The model under review builds one solid part; all positions refer to its coordinate system, in mm. A direction names the side the tool comes from. Coordinates: 2 decimals unless noted, no trailing zeros. Write each loop counter-clockwise with the first axis right and the second up, starting at its lowest first coordinate (ties: lowest second). Pieces come first, ordered by that corner, then holes.
1) For P1, Ø3.5, axis at x = 171.5, z = 59.5, coming from the +Y side; P2, Ø4, axis at x = 127.5, y = 41, coming from the -Z side; P3, Ø2.5, axis at x = 55, y = 4.5, coming from the -Z side, all flat-tipped, find the tip position at first contact; note any pin that passes through.
2) For line 1 (Z direction, x = 172, y = 4.55); line 2 (X direction, y = 112, z = 12.5); line 3 (Z direction, x = 150, y = 63.5), list the stretches that pass through material, from the lowest coordinate up.
3) Add section C-C, the plane z = 107. State the section outline as (x, y) points.
4) Add section B-B, the plane y = 11. State the section outline as (x, z) points.
5) Machinability: for faces 4 (the flat face through (165, 5.5, 60)), 5 (the flat face through (110, 2.5, 60)), 6 (the flat face through (111, 2, 0)), 7 (the flat face through (224, 58, 61)), 8 (the flat face through (110.47, 137.92, 18.76)), which of the approach directions +Z, -Z, +X, -X, +Y, -Y give a long, thin tool a straight path to every point of the face, cutting with its end or side? Answer none if there is none.
6) Mouldability with a two-part tool opening along Y and no side actions: class faces 1 (the flat face through (110, 41, 120)), 2 (the flat face through (2.5, 59, 60)), 3 (the flat face through (60, 5.5, 30)) as released by +Y, released by -Y, zero draft, split by the parting line, or undercut.
7) Add section A-A, the plane x = 100. State the section outline as (y, z) points.
8) Add section D-D, the plane x = 14. State the section outline as (y, z) points.
from build123d import *

# Parameters (mm, degrees)
F1_DEPTH = 224
F2_T     = -2.5
F3_W     = 164
F3_H     = 80
F4_DEPTH = 6
F5_W     = 20
F5_H     = 5
F5_R     = 1.7
F6_DEPTH = 3


with BuildPart() as f1:
    # F0 (on Right) → F1 (new body)
    with BuildSketch(Plane.YZ):
        Polygon((0, 120), (0, 0), (152.1110255093, 0), (80, 120), align=None)
    extrude(amount=F1_DEPTH)

    # F2
    f2_openings = [f1.faces().sort_by_distance(p)[0] for p in [
        (112, 76.055513, 0),
    ]]
    offset(amount=F2_T, openings=f2_openings, kind=Kind.INTERSECTION)

    # F3 (on face) → F4 (cut)
    with BuildSketch(Plane(origin=(0, 111.7550391497, 67.1564206576), x_dir=(-1, 0, 0), z_dir=(0, 0.8571428571, 0.5150787536))):
        with Locations((-112, -8.3491574339)):
            Rectangle(F3_W, F3_H)
    extrude(amount=-F4_DEPTH, mode=Mode.SUBTRACT)

    # F5 (on face) → F6 (join)
    with BuildSketch(Plane(origin=(0, 2.5, 0), x_dir=(-1, 0, 0), z_dir=(0, 1, 0))):
        with Locations((-164.5, 30)):
            Rectangle(F5_W, F5_H)
        with Locations((-172, 30)):
            Circle(F5_R, mode=Mode.SUBTRACT)
        with Locations((-164.5, 60)):
            Rectangle(F5_W, F5_H)
        with Locations((-172, 60)):
            Circle(F5_R, mode=Mode.SUBTRACT)
        with Locations((-59.5, 30)):
            Rectangle(F5_W, F5_H)
        with Locations((-52, 30)):
            Circle(F5_R, mode=Mode.SUBTRACT)
        with Locations((-59.5, 60)):
            Rectangle(F5_W, F5_H)
        with Locations((-52, 60)):
            Circle(F5_R, mode=Mode.SUBTRACT)
    extrude(amount=F6_DEPTH)


solid = f1.part
Geometry results:
1. P1: stops at y = 5.5
1. P2: stops at z = 117.5
1. P3: stops at z = 27.5
2. line 1: z = 27.5 to 28.3, 31.7 to 32.5, 57.5 to 58.3, 61.7 to 62.5, 117.5 to 120
2. line 2: x = 0 to 2.5, 221.5 to 224
2. line 3: z = 117.5 to 120
3. outline: (0, 0) - (224, 0) - (224, 87.81) - (0, 87.81) - close; hole (2.5, 2.5) - (221.5, 2.5) - (221.5, 84.9) - (2.5, 84.9) - close
4. outline: (0, 0) - (2.5, 0) - (2.5, 117.5) - (221.5, 117.5) - (221.5, 0) - (224, 0) - (224, 120) - (0, 120) - close
5. face 4: -Z, +Y
5. face 5: none
5. face 6: -Z, +X, -X, +Y, -Y
5. face 7: +Z, -Z, +X, +Y, -Y
5. face 8: -Z
6. face 1: zero draft
6. face 2: undercut
6. face 3: released by +Y
7. outline: (0, 0) - (2.5, 0) - (2.5, 117.5) - (78.59, 117.5) - (93.31, 93) - (95.45, 94.29) - (80, 120) - (0, 120) - close; (134.52, 24.43) - (149.19, 0) - (152.11, 0) - (136.66, 25.71) - close
8. outline: (0, 0) - (2.5, 0) - (2.5, 117.5) - (78.59, 117.5) - (149.19, 0) - (152.11, 0) - (80, 120) - (0, 120) - close
